Could you check a few things on this model? Use its own coordinates, in mm. A direction names the side the tool comes from. Give positions to 0.01 mm unless a question says otherwise; leave off trailing zeros. Write each loop counter-clockwise with the first axis right and the second up, starting at its lowest first coordinate (ties: lowest second). Pieces come first, ordered by that corner, then holes. Notation, with made-up numbers: (14, -20) - (48, -20) arc R20 ccw to (48, -7) - close; hole circle Ø11 at (75.5, 85). An arc over 180 degrees is marked (long way). Answer in a Markdown table with one row per item.
from build123d import *

# Parameters (mm, degrees)
SKETCH1_W           = 66
SKETCH1_H           = 50
SKETCH1_R           = 1
BOSS_EXTRUDE1_DEPTH = 5
SKETCH2_R           = 1
CUT_EXTRUDE1_DEPTH  = 388.996134001
SKETCH3_R           = 1
SKETCH3_W           = 20
SKETCH3_H           = 5
CUT_EXTRUDE2_DEPTH  = 388.996134001
CUT_EXTRUDE3_DEPTH  = 388.996134001


with BuildPart() as part:
    # Sketch1 → Boss-Extrude1 (new body)
    # profile 1 of 3: a face of its own
    with BuildSketch(Plane.XY):
        with Locations((-33, 85)):
            Rectangle(SKETCH1_W, SKETCH1_H)
    # profile 2 of 3: a face of its own
    with BuildSketch(Plane.XY):
        Polygon((0, 60), (0, 0), (180, 0), (180, 60), (180, 110), (180, 300), (130, 300), (130, 150), (50, 150), (50, 300), (0, 300), (0, 110), align=None)
        with Locations((19, 117.5)):
            Circle(SKETCH1_R, mode=Mode.SUBTRACT)
        with Locations((38, 117.5)):
            Circle(SKETCH1_R, mode=Mode.SUBTRACT)
        with Locations((19, 134)):
            Circle(SKETCH1_R, mode=Mode.SUBTRACT)
        with Locations((38, 134)):
            Circle(SKETCH1_R, mode=Mode.SUBTRACT)
        with Locations((142, 117.5)):
            Circle(SKETCH1_R, mode=Mode.SUBTRACT)
        with Locations((161, 117.5)):
            Circle(SKETCH1_R, mode=Mode.SUBTRACT)
        with Locations((142, 134)):
            Circle(SKETCH1_R, mode=Mode.SUBTRACT)
        with Locations((161, 134)):
            Circle(SKETCH1_R, mode=Mode.SUBTRACT)
    # profile 3 of 3: a face of its own
    with BuildSketch(Plane.XY):
        with Locations((213, 85)):
            Rectangle(SKETCH1_W, SKETCH1_H)
    extrude(amount=BOSS_EXTRUDE1_DEPTH)

    # Sketch2 → Cut-Extrude1 (cut, through all)
    with BuildSketch(Plane.XY.offset(5)):
        with Locations((-58, 103)):
            Circle(SKETCH2_R)
        with Locations((-58, 67)):
            Circle(SKETCH2_R)
        with Locations(Location((238, 67, 0), (0, 0, 180))):
            Circle(SKETCH2_R)
        with Locations(Location((238, 103, 0), (0, 0, 180))):
            Circle(SKETCH2_R)
    extrude(amount=-CUT_EXTRUDE1_DEPTH, mode=Mode.SUBTRACT)

    # Sketch3 → Cut-Extrude2 (cut, through all)
    with BuildSketch(Plane.XY.offset(5)):
        with Locations((19, 77)):
            Circle(SKETCH3_R)
        with Locations((19, 99.5)):
            Circle(SKETCH3_R)
        with Locations(Location((161, 77, 0), (0, 0, 180))):
            Circle(SKETCH3_R)
        with Locations(Location((161, 99.5, 0), (0, 0, 180))):
            Circle(SKETCH3_R)
        with Locations((-6, 90)):
            Rectangle(SKETCH3_W, SKETCH3_H)
        with Locations((186, 90)):
            Rectangle(SKETCH3_W, SKETCH3_H)
    extrude(amount=-CUT_EXTRUDE2_DEPTH, mode=Mode.SUBTRACT)

    # Sketch4 → Cut-Extrude3 (cut, through all)
    with BuildSketch(Plane.XY.offset(5)):
        Polygon((180, 60), (130, 60), (130, 150), (65.062754068, 311.897276324), (-51.051297303, 321.248743549), (-107.939389585, -9.16976505), (175.332138424, -20.859099081), (198.321162017, 8.753880463), align=None)
    extrude(amount=-CUT_EXTRUDE3_DEPTH, mode=Mode.SUBTRACT)


solid = part.part
1) Will these pins go through, and if not, where does the flat tip stop? P1, Ø1.5, axis at y = 223, z = 3.5, coming from the +X side; P2, Ø1.5, axis at x = 186.5, z = 1.5, coming from the +Y side.
Check values:
| item | result |
|---|---|
| P1 | stops at x = 180 |
| P2 | stops at y = 110 |
2) Imagine slicing it at A-A (x = 191). List the corners of the cut face in (y, z) for me.
Check values:
| item | result |
|---|---|
| outline | (60, 0) - (87.5, 0) - (87.5, 5) - (60, 5) - close; (92.5, 0) - (110, 0) - (110, 5) - (92.5, 5) - close |
3) Imagine slicing it at B-B (z = 2.75). State how many separate pieces and enclosed holes the cut face has, then the cut area to 3 significant figures.
Check values:
| item | result |
|---|---|
| separate pieces | 1 |
| enclosed holes | 9 |
| area | 15,200 mm2 |
4) Imagine slicing it at C-C (y = 190). List the corners of the cut face in (x, z) for me, then the cut area to 3 significant figures.
Check values:
| item | result |
|---|---|
| outline | (130, 0) - (180, 0) - (180, 5) - (130, 5) - close |
| area | 250 mm2 |
5) Imagine slicing it at D-D (x = 219). List the corners of the cut face in (y, z) for me, then the cut area to 3 significant figures.
Check values:
| item | result |
|---|---|
| outline | (60, 0) - (110, 0) - (110, 5) - (60, 5) - close |
| area | 250 mm2 |
6) We'd pull the mould along Y, two halves only. Please class faces 1 (the face through (213, 110, 2)), 2 (the face through (180, 204, 2)), 3 (the face through (186, 87.5, 3)): +Y half, -Y half, draft (parallel to the pull), parting line (faces both ways), or undercut.
Check values:
| item | result |
|---|---|
| face 1 | +Y half |
| face 2 | draft |
| face 3 | undercut |
7) If I drill on line 1 (Y direction, x = 142, z = 3.75); line 2 (Y direction, x = 161, z = 1.45); line 3 (X direction, y = 117.5, z = 3.65), over which ranges is the centre line in solid material (lowest first)?
Check values:
| item | result |
|---|---|
| line 1 | y = 60 to 116.5, 118.5 to 133, 135 to 300 |
| line 2 | y = 60 to 76, 78 to 98.5, 100.5 to 116.5, 118.5 to 133, 135 to 300 |
| line 3 | x = 130 to 141, 143 to 160, 162 to 180 |
8) On a 3-axis mill with a long thin cutter (end or side, diameter ignored), from which of +Z, -Z, +X, -X, +Y, -Y can I reach the whole of each face in a straight line? I mean faces 4 (the face through (176, 90, 3)), 5 (the face through (161, 155, 5)). Say none if no direction works.
Check values:
| item | result |
|---|---|
| face 4 | +Z, -Z |
| face 5 | +Z, +X, -X, +Y, -Y |
